Source: CAD feature listing. Evaluate the final solid. Frame: model axes, mm. A direction names the side the tool comes from. Give positions to 0.01 mm unless a question says otherwise; leave off trailing zeros. Loops run counter-clockwise (first coordinate to the right, second up) from the corner with the lowest first, then second, coordinate; pieces in that order, holes last. Notation, with made-up numbers: (22.5, -22) -> (35.5, -22) arc R29 ccw to (35.5, 7) -> close; hole circle Ø8 at (55, -22). An arc over 180 degrees is marked (long way). Return JSON: item names as keys, results as strings. Group by question number.
(1) Cut plane C-C on y = -313.5. Return loops of the section in (x, z).
(2) Access query for faces 1 (the face through (431.7, -177, 250)), 2 (the face through (-304, -75, 0)), 3 (the face through (572, -18, 0)), 4 (the face through (431.7, -477, 98)), 5 (the face through (-537.3, -75, 0)). Directions: +Z, -Z, +X, -X, +Y, -Y. A direction counts if a zero-diameter tool reaches every point of the face in a straight line with its end or side. Return the directions, or none.
(3) Draft query along Y for faces 6 (the face through (467, -213, 236)), 7 (the face through (-451, -18, 335.4)). Return one class per face: released by +Y, released by -Y, zero draft, split by the parting line, or undercut.
(4) Cut plane A-A on x = 77.5. Return loops of the section in (y, z).
(5) Cut plane B-B on z = 220.5. Give the number of separate pieces and of enclosed holes in the cut face, then the cut area to 3 significant figures.
(6) Pin query (flat end, axial travel): pin 1 (23 mm diameter, centred on x = 96.5, y = -23, fed in from +Z); pin 2 (16.5 mm diameter, centred on y = -99.8, z = 0, fed in from -X); pin 3 (10 mm diameter, centred on x = -34.5, z = 187.5, fed in from +Y); pin 4 (11.5 mm diameter, centred on y = -475, z = 119, fed in from -X). Return the tip coordinate at first contact, or that it passes through.
(7) Cut plane D-D on x = 491. Return loops of the section in (y, z).
(8) Ray query, line 1 (X direction, y = -122.5, z = 273); line 2 (Y direction, x = 532, z = 0); line 3 (Z direction, x = -437.5, y = -461.5). Return the intervals inside material, ascending. Write a range as from..to.
```python
from build123d import *

# Parameters (mm, degrees)
SKETCH1_W            = 1150
SKETCH1_H            = 56
BOSS_EXTRUDE1_DEPTH  = 35
SKETCH2_W            = 38.3
SKETCH2_H            = 35
BOSS_EXTRUDE2_DEPTH  = 268
BOSS_EXTRUDE3_DEPTH  = 38.3
BOSS_EXTRUDE4_DEPTH  = 38.3
SKETCH5_W            = 38.3
SKETCH5_H            = 39.42449842
BOSS_EXTRUDE5_DEPTH  = 38.5
BOSS_EXTRUDE6_DEPTH  = 901.7
SKETCH8_W            = 38.3
SKETCH8_H            = 38.5
BOSS_EXTRUDE7_DEPTH  = 90
SHELL2_START         = -467
SHELL2_OUTLINE_W     = 29
SHELL2_OUTLINE_H     = 50
SHELL2_DEPTH         = 934
SHELL2_2_DEPTH       = 32.3
SHELL2_START_2       = 434.7
SHELL2_3_DEPTH       = 32.3
SHELL2_START_3       = -575
SHELL2_4_OUTLINE_W   = 29
SHELL2_4_OUTLINE_H   = 50
SHELL2_4_DEPTH       = 1147
SKETCH13_W           = 50
SKETCH13_H           = 29
BOSS_EXTRUDE8_DEPTH  = 3
SKETCH14_R           = 4.75
CUT_EXTRUDE1_DEPTH   = 1390
SKETCH15_W           = 8.185813993
SKETCH15_H           = 78
SKETCH15_W_2         = 6
BOSS_EXTRUDE10_DEPTH = 56
FILLET2_R            = 4
SKETCH16_R           = 6.3
CUT_EXTRUDE2_DEPTH   = 1390


# Read off the part's stored shape, not the designer's step: Shell2
with BuildPart() as part:
    # Sketch1 → Boss-Extrude1 (new body)
    with BuildSketch(Plane(origin=(0, 0, 0), x_dir=(1, 0, 0), z_dir=(0, 1, 0))):
        Rectangle(SKETCH1_W, SKETCH1_H)
    extrude(amount=-BOSS_EXTRUDE1_DEPTH)

    # Sketch2 → Boss-Extrude2 (add)
    with BuildSketch(Plane.XY.offset(28)):
        with Locations((-450.85, -17.5)):
            Rectangle(SKETCH2_W, SKETCH2_H)
        with Locations((450.85, -17.5)):
            Rectangle(SKETCH2_W, SKETCH2_H)
    extrude(amount=BOSS_EXTRUDE2_DEPTH)

    # Sketch3 → Boss-Extrude3 (add)
    with BuildSketch(Plane.ZY.offset(470)):
        Polygon((296, -35), (142.090935503, -457.861679354), (181.515376734, -457.794527623), (335.4, -35), (335.4, 0), (296, 0), align=None)
    extrude(amount=-BOSS_EXTRUDE3_DEPTH)

    # Sketch4 → Boss-Extrude4 (add)
    with BuildSketch(Plane.ZY.offset(-431.7)):
        Polygon((296, 0), (335.4, 0), (335.4, -35), (181.515376734, -457.794527623), (142.090935503, -457.861679354), (296, -35), align=None)
    extrude(amount=-BOSS_EXTRUDE4_DEPTH)

    # Sketch5 → Boss-Extrude5 (add)
    with BuildSketch(Plane(origin=(0, -458.102374067, 0.780286699), x_dir=(1, 0, 0), z_dir=(0, -0.9999985493842727, 0.0017032995480483616))):
        with Locations((450.85, 161.023103003)):
            Rectangle(SKETCH5_W, SKETCH5_H)
    extrude(amount=BOSS_EXTRUDE5_DEPTH)

    # Sketch6 → Boss-Extrude6 (add)
    with BuildSketch(Plane.ZY.offset(-431.7)):
        Polygon((142.090935503, -457.861679354), (181.515376734, -457.794527623), (181.580953767, -496.294471775), (142.156512536, -496.361623505), align=None)
    extrude(amount=BOSS_EXTRUDE6_DEPTH)

    # Sketch8 → Boss-Extrude7 (add)
    with BuildSketch(Plane(origin=(0, 0.240694713, 141.310648805), x_dir=(-1, 0, 0), z_dir=(0, -0.0017032995480483616, -0.9999985493842727))):
        with Locations((-450.85, -477.353038599)):
            Rectangle(SKETCH8_W, SKETCH8_H)
        with Locations((450.85, -477.353038599)):
            Rectangle(SKETCH8_W, SKETCH8_H)
    extrude(amount=BOSS_EXTRUDE7_DEPTH)

    # Shell2 outline → Shell2 (cut)
    with BuildSketch(Plane.YZ.offset(SHELL2_START)):
        Polygon((-493.356517958, 145.151398286), (-460.856565103, 145.09604105), (-460.79963317, 178.520490985), (-493.299586025, 178.57584822), align=None)
        with Locations((-17.5, 0)):
            Rectangle(SHELL2_OUTLINE_W, SHELL2_OUTLINE_H)
    extrude(amount=SHELL2_DEPTH, mode=Mode.SUBTRACT)

    # Shell2 2 outline → Shell2 2 (cut)
    with BuildSketch(Plane.YZ.offset(SHELL2_START)):
        Polygon((-460.79963317, 178.520490985), (-460.856565103, 145.09604105), (-493.356517958, 145.151398286), (-493.509814917, 55.151528841), (-461.009862062, 55.096171606), (-460.858103494, 144.192859625), (-32, 300.28444402), (-32, 25), (-3, 25), (-3, 332.4), (-34.471019058, 332.4), (-457.268022568, 178.514475585), align=None)
    extrude(amount=SHELL2_2_DEPTH, mode=Mode.SUBTRACT)

    # Shell2 3 outline → Shell2 3 (cut)
    with BuildSketch(Plane.YZ.offset(SHELL2_START_2)):
        Polygon((-460.79963317, 178.520490985), (-460.856565103, 145.09604105), (-493.356517958, 145.151398286), (-493.509814917, 55.151528841), (-461.009862062, 55.096171606), (-460.858103494, 144.192859625), (-32, 300.28444402), (-32, 25), (-3, 25), (-3, 332.4), (-34.471019058, 332.4), (-457.268022568, 178.514475585), align=None)
    extrude(amount=SHELL2_3_DEPTH, mode=Mode.SUBTRACT)

    # Shell2 4 outline → Shell2 4 (cut)
    with BuildSketch(Plane.YZ.offset(SHELL2_START_3)):
        with Locations((-17.5, 0)):
            Rectangle(SHELL2_4_OUTLINE_W, SHELL2_4_OUTLINE_H)
    extrude(amount=SHELL2_4_DEPTH, mode=Mode.SUBTRACT)

    # Sketch13 → Boss-Extrude8 (add)
    with BuildSketch(Plane.ZY.offset(575)):
        with Locations((0, -17.5)):
            Rectangle(SKETCH13_W, SKETCH13_H)
    extrude(amount=-BOSS_EXTRUDE8_DEPTH)

    # Sketch14 → Cut-Extrude1 (cut)
    with BuildSketch(Plane(origin=(470, 0, 0), x_dir=(0, 0, -1), z_dir=(1, 0, 0))):
        with Locations((-74.873854575, -477.264948389)):
            Circle(SKETCH14_R)
    extrude(amount=-CUT_EXTRUDE1_DEPTH, mode=Mode.SUBTRACT)

    # Sketch15 → Boss-Extrude10 (add)
    with BuildSketch(Plane(origin=(0, 0, -28), x_dir=(-1, 0, 0), z_dir=(0, 0, -1))):
        with Locations((308.092906997, -74)):
            Rectangle(SKETCH15_W, SKETCH15_H)
        with Locations((534.3, -74)):
            Rectangle(SKETCH15_W_2, SKETCH15_H)
        with Locations((-534.3, -74)):
            Rectangle(SKETCH15_W_2, SKETCH15_H)
        with Locations((-308.092906997, -74)):
            Rectangle(SKETCH15_W, SKETCH15_H)
    extrude(amount=-BOSS_EXTRUDE10_DEPTH)

    # Fillet2
    fillet2_edges = [part.edges().sort_by_distance(p)[0] for p in [
        (-308.092906997, -113, -28),
        (-308.092906997, -113, 28),
        (-534.3, -113, -28),
        (-534.3, -113, 28),
        (534.3, -113, -28),
        (534.3, -113, 28),
        (308.092906997, -113, -28),
        (308.092906997, -113, 28),
    ]]
    fillet(fillet2_edges, radius=FILLET2_R)

    # Sketch16 → Cut-Extrude2 (cut)
    with BuildSketch(Plane(origin=(537.3, 0, 0), x_dir=(0, 0, -1), z_dir=(1, 0, 0))):
        with Locations((0, -99.8)):
            Circle(SKETCH16_R)
    extrude(amount=-CUT_EXTRUDE2_DEPTH, mode=Mode.SUBTRACT)


solid = part.part
```
Answers:
{
 "1": {"outline": "(-470, 194.63) -> (-431.7, 194.63) -> (-431.7, 234.03) -> (-470, 234.03) -> close; (431.7, 194.63) -> (470, 194.63) -> (470, 234.03) -> (431.7, 234.03) -> close; hole (-467, 197.83) -> (-434.7, 197.83) -> (-434.7, 230.84) -> (-467, 230.84) -> close; hole (434.7, 197.83) -> (467, 197.83) -> (467, 230.84) -> (434.7, 230.84) -> close"},
 "2": {"face 1": "+Z, +Y", "face 2": "+Z, -Z, -Y", "face 3": "none", "face 4": "-Z, +Y, -Y", "face 5": "+Z, -Z, -X, -Y"},
 "3": {"face 6": "undercut", "face 7": "zero draft"},
 "4": {"outline": "(-496.36, 142.16) -> (-457.86, 142.09) -> (-457.79, 181.52) -> (-496.29, 181.58) -> close; (-35, -28) -> (0, -28) -> (0, 28) -> (-35, 28) -> close; hole (-493.36, 145.15) -> (-460.86, 145.1) -> (-460.8, 178.52) -> (-493.3, 178.58) -> close; hole (-32, -25) -> (-3, -25) -> (-3, 25) -> (-32, 25) -> close"},
 "5": {"separate pieces": "4", "enclosed holes": "4", "area": "3,240 mm²"},
 "6": {"pin 1": "z = 28", "pin 2": "x = -537.3", "pin 3": "through", "pin 4": "x = -470"},
 "7": {"outline": "(-35, -28) -> (0, -28) -> (0, 28) -> (-35, 28) -> close; hole (-32, -25) -> (-3, -25) -> (-3, 25) -> (-32, 25) -> close"},
 "8": {"line 1": "-470..-467, -434.7..-431.7, 431.7..434.7, 467..470", "line 2": "-113..-106.1, -93.5..-32, -3..0", "line 3": "52.1..55.1, 178.52..181.52"}
}
